Could you check a few things on this model? Use its own coordinates, in mm. Give positions to 0.01 mm unless a question says otherwise; leave off trailing zeros. Write each loop counter-clockwise with the first axis right and the second up, starting at its lowest first coordinate (ties: lowest second). Pieces come first, ordered by that corner, then holes. Notation, with made-up numbers: (42.25, -26) - (99.25, -26) arc R6 ccw to (99.25, -20) - close; hole circle Ø2 at (76, 58.5). An arc over 180 degrees is marked (long way). Write item = value, one per line.
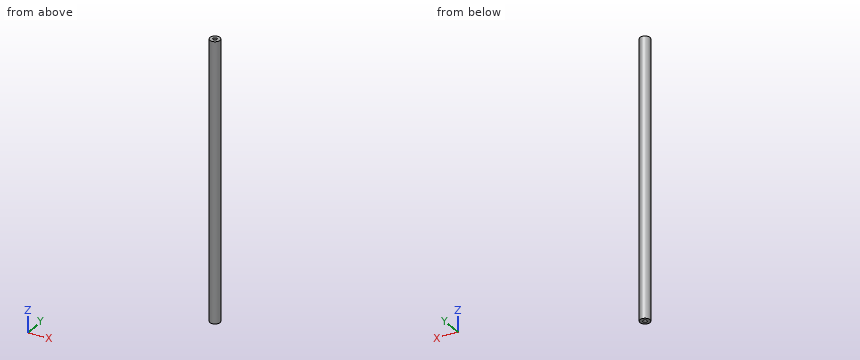
from build123d import *

# Parameters (mm, degrees)
SKETCH1_R           = 6.35
BOSS_EXTRUDE1_DEPTH = 177.8
SKETCH3_R           = 2.4892
CUT_EXTRUDE1_DEPTH  = 19.05


with BuildPart() as part:
    # Sketch1 → Boss-Extrude1 (new, symmetric)
    with BuildSketch(Plane.XY):
        Circle(SKETCH1_R)
    extrude(amount=BOSS_EXTRUDE1_DEPTH, both=True)

    # Sketch3 → Cut-Extrude1 (cut)
    with BuildSketch(Plane.XY.offset(177.8)):
        Circle(SKETCH3_R)
    cut_extrude1 = extrude(amount=-CUT_EXTRUDE1_DEPTH, mode=Mode.SUBTRACT)

    # Mirror1: Cut-Extrude1 across plane
    add(cut_extrude1.mirror(Plane.XY), mode=Mode.SUBTRACT)


solid = part.part
1. If we section it at C-C, the plane z = 78: Please give me the cut outline in (x, y).
Filled sheet:
outline = circle Ø12.7 at (0, 0)
2. I need wall thicknesses on line 1 (Y direction, x = 0, z = 167.25); line 2 (Z direction, x = -0.25, y = 0.75); line 3 (Y direction, x = 0.5, z = 61). Which ranges of each line are inside material? Lowest first, please.
Filled sheet:
line_1 = -6.35 to -2.49, 2.49 to 6.35
line_2 = -158.75 to 158.75
line_3 = -6.33 to 6.33
3. For pin 1 (6 mm diameter, centred on x = -1, z = -75.5, fed in from -Y); pin 2 (3 mm diameter, centred on y = -3, z = 51.5, fed in from -X); pin 3 (4.5 mm diameter, centred on x = 0, y = 0, fed in from +Z), each with a flat end and sliding along its axis, tell me the tip position at first contact or that it passes through.
Filled sheet:
pin_1 = -6.35
pin_2 = -6.17
pin_3 = 158.75
4. If we section it at A-A, the plane x = 0: Please give me the cut outline in (y, z).
Filled sheet:
outline = (-6.35, -177.8) - (-2.49, -177.8) - (-2.49, -158.75) - (2.49, -158.75) - (2.49, -177.8) - (6.35, -177.8) - (6.35, 177.8) - (2.49, 177.8) - (2.49, 158.75) - (-2.49, 158.75) - (-2.49, 177.8) - (-6.35, 177.8) - close
